Work out the finished part from the listing and answer in its coordinate system (mm). Face numbers are marked on the shaded views. A direction names the side the tool comes from. Coordinates: 2 decimals unless noted, no trailing zeros. Loops run counter-clockwise (first coordinate to the right, second up) from the corner with the lowest first, then second, coordinate; pieces in that order, holes last. Notation, with made-up numbers: (34, -29) -> (39, -29) arc R31 cw to (39, 9) -> close; hole circle Ø1 at (23.25, 77.25). An arc over 180 degrees is marked (long way). One line per question, with ' | ' between items.
```python
from build123d import *

# Parameters (mm, degrees)
F1_DEPTH  = 20
F2_R      = 11.01
F3_DEPTH  = 10
F4_R      = 3.01
F5_DEPTH  = 15
F6_R      = 3.01
F7_DEPTH  = 15
F8_R      = 2.01
F9_DEPTH  = 23.251
F10_R     = 2.01
F11_DEPTH = 23.251


with BuildPart() as f1:
    # F0 (on Top) → F1 (new body)
    with BuildSketch(Plane.XY):
        with BuildLine():
            Line((0, 50), (0, 0))
            Line((0, 0), (26.933724, 0))
            Line((26.933724, 0), (38.25, 0))
            Line((38.25, 0), (38.25, 10))
            ThreePointArc((38.25, 10), (53.25, 25), (38.25, 40))
            Line((38.25, 40), (38.25, 50))
            Line((38.25, 50), (0, 50))
        make_face()
    extrude(amount=F1_DEPTH)

    # F2 (on face) → F3 (cut)
    with BuildSketch(Plane.XY.offset(20)):
        with Locations((38.25, 25)):
            Circle(F2_R)
    extrude(amount=-F3_DEPTH, mode=Mode.SUBTRACT)

    # F4 (on face) → F5 (cut)
    with BuildSketch(Plane.YZ.offset(38.25)):
        with Locations((45, 10)):
            Circle(F4_R)
    extrude(amount=-F5_DEPTH, mode=Mode.SUBTRACT)

    # F6 (on face) → F7 (cut)
    with BuildSketch(Plane.YZ.offset(38.25)):
        with Locations((5, 10)):
            Circle(F6_R)
    extrude(amount=-F7_DEPTH, mode=Mode.SUBTRACT)

    # F8 (on face) → F9 (cut, through all)
    with BuildSketch(Plane.YZ.offset(23.25)):
        with Locations((5, 10)):
            Circle(F8_R)
    extrude(amount=-F9_DEPTH, mode=Mode.SUBTRACT)

    # F10 (on face) → F11 (cut, through all)
    with BuildSketch(Plane.YZ.offset(23.25)):
        with Locations((45, 10)):
            Circle(F10_R)
    extrude(amount=-F11_DEPTH, mode=Mode.SUBTRACT)


solid = f1.part
```
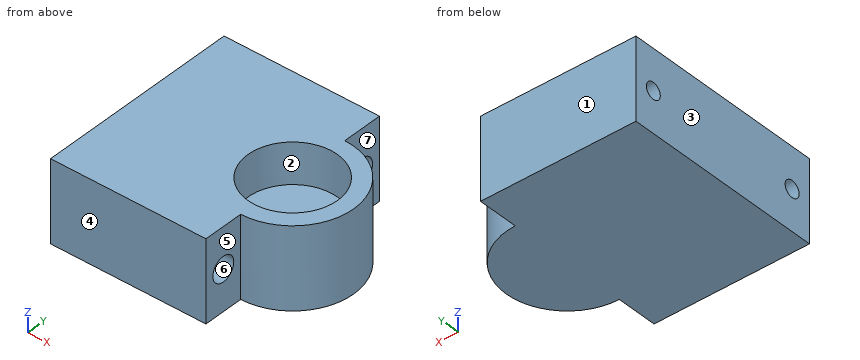
1) Find the intervals of material crossed by line 1 along Z through (x, y) = (32, 45); line 2 along Z through (x, y) = (11, 5); line 3 along X through (y, z) = (24.5, 11.25), in increasing order.
Check values:
line 1: z = 0 to 6.99, 13.01 to 20 | line 2: z = 0 to 7.99, 12.01 to 20 | line 3: x = 0 to 27.25, 49.25 to 53.24
2) Find section B-B (x = 9.5). Write down the section's boundary in (y, z), plus the area to 3 significant figures.
Check values:
outline: (0, 0) -> (50, 0) -> (50, 20) -> (0, 20) -> close; hole circle Ø4.02 at (5, 10); hole circle Ø4.02 at (45, 10) | area: 975 mm^2
3) The mould has two halves that part along Y. Classify the marked faces 1, 2, 3 and 4: released by +Y, released by -Y, zero draft, split by the parting line, or undercut.
Check values:
face 1: released by +Y | face 2: undercut | face 3: zero draft | face 4: released by -Y
4) Find section D-D (y = 25). Write down the section's boundary in (x, z), plus the area to 3 significant figures.
Check values:
outline: (0, 0) -> (53.25, 0) -> (53.25, 20) -> (49.26, 20) -> (49.26, 10) -> (27.24, 10) -> (27.24, 20) -> (0, 20) -> close | area: 845 mm^2
5) For the marked faces 5, 6 and 7, determine the directions among +Z, -Z, +X, -X, +Y, -Y from which every point of the face is accessible in a straight line to the end or side of a thin tool.
Check values:
face 5: +Z, -Z, +X, -Y | face 6: +X | face 7: +Z, -Z, +X, +Y
6) Find section C-C (z = 15.5). Write down the section's boundary in (x, y).
Check values:
outline: (0, 0) -> (38.25, 0) -> (38.25, 10) arc R15 ccw to (38.25, 40) -> (38.25, 50) -> (0, 50) -> close; hole circle Ø22.02 at (38.25, 25)
7) Flat-ended cylindrical pins translate along their axes: pin 1 (6.5 mm diameter, centred on y = 45.5, z = 10, fed in from +X); pin 2 (5 mm diameter, centred on y = 5, z = 10, fed in from +X). Find the tip coordinate at first contact, or state that the pin passes through.
Check values:
pin 1: stops at x = 38.25 | pin 2: stops at x = 23.25
8) Find section A-A (y = 5). Write down the section's boundary in (x, z).
Check values:
outline: (0, 0) -> (38.25, 0) -> (38.25, 6.99) -> (23.25, 6.99) -> (23.25, 7.99) -> (0, 7.99) -> close; (0, 12.01) -> (23.25, 12.01) -> (23.25, 13.01) -> (38.25, 13.01) -> (38.25, 20) -> (0, 20) -> close
